Verification items for the finished model (mm, model axes). A direction names the side the tool comes from. Coordinates: 2 decimals unless noted, no trailing zeros. Write each loop counter-clockwise with the first axis right and the second up, starting at its lowest first coordinate (ties: lowest second). Pieces come first, ordered by that corner, then holes. Notation, with made-up numbers: (11, 59.5) - (60, 59.5) arc R12 ccw to (60, 75.5) - close; hole circle Ø11 at (-5.75, -7). An arc over 180 degrees is marked (long way). Use CSV: the item, a comma, the result in double quotes. Start each with the question number.
```python
from build123d import *

# Parameters (mm, degrees)
BOSS_EXTRUDE1_DEPTH = 2.1
SKETCH2_W           = 57.36
SKETCH2_H           = 70
BOSS_EXTRUDE2_DEPTH = 7
SKETCH3_W           = 53.36
SKETCH3_H           = 66
CUT_EXTRUDE1_DEPTH  = 7
SKETCH4_R           = 1.5
CUT_EXTRUDE2_DEPTH  = 2.1
SKETCH6_W           = 40.39
SKETCH6_H           = 2
CUT_EXTRUDE3_DEPTH  = 9.1
BOSS_EXTRUDE3_DEPTH = 9.1
BOSS_EXTRUDE4_DEPTH = 2.1


with BuildPart() as part:
    # Sketch1 → Boss-Extrude1 (new body)
    with BuildSketch(Plane(origin=(0, 0, 0), x_dir=(1, 0, 0), z_dir=(0, 1, 0))):
        Polygon((28.68, 0), (28.68, -8), (28.68, -78), (-28.68, -78), (-28.68, 0), align=None)
    extrude(amount=BOSS_EXTRUDE1_DEPTH)

    # Sketch2 → Boss-Extrude2 (add)
    with BuildSketch(Plane(origin=(0, 2.1, 0), x_dir=(1, 0, 0), z_dir=(0, 1, 0))):
        with Locations((0, -43)):
            Rectangle(SKETCH2_W, SKETCH2_H)
    extrude(amount=BOSS_EXTRUDE2_DEPTH)

    # Sketch3 → Cut-Extrude1 (cut)
    with BuildSketch(Plane(origin=(0, 9.1, 0), x_dir=(1, 0, 0), z_dir=(0, 1, 0))):
        with Locations((0, -43)):
            Rectangle(SKETCH3_W, SKETCH3_H)
    extrude(amount=-CUT_EXTRUDE1_DEPTH, mode=Mode.SUBTRACT)

    # Sketch4 → Cut-Extrude2 (cut)
    with BuildSketch(Plane(origin=(0, 2.1, 0), x_dir=(1, 0, 0), z_dir=(0, 1, 0))):
        with Locations((24.5, -4)):
            Circle(SKETCH4_R)
        with Locations((-24.5, -4)):
            Circle(SKETCH4_R)
    extrude(amount=-CUT_EXTRUDE2_DEPTH, mode=Mode.SUBTRACT)

    # Sketch6 → Cut-Extrude3 (cut)
    with BuildSketch(Plane(origin=(0, 9.1, 0), x_dir=(1, 0, 0), z_dir=(0, 1, 0))):
        with Locations((-6.485, -77)):
            Rectangle(SKETCH6_W, SKETCH6_H)
    extrude(amount=-CUT_EXTRUDE3_DEPTH, mode=Mode.SUBTRACT)

    # Sketch5 → Boss-Extrude3 (add)
    with BuildSketch(Plane(origin=(0, 9.1, 0), x_dir=(1, 0, 0), z_dir=(0, 1, 0))):
        Polygon((-26.68, -76), (-24.14, -76), (-21.6, -78.54), (11.17, -78.54), (13.71, -76), (14.538427125, -76), (14.538427125, -78), (11.998427125, -80.54), (-22.428427125, -80.54), (-24.968427125, -78), (-26.68, -78), align=None)
    extrude(amount=-BOSS_EXTRUDE3_DEPTH)

    # Sketch7 → Boss-Extrude4 (add)
    with BuildSketch(Plane.XZ):
        Polygon((13.71, 76), (-24.14, 76), (-21.6, 78.54), (11.17, 78.54), align=None)
    extrude(amount=-BOSS_EXTRUDE4_DEPTH)


solid = part.part
```
Q1. Gauge pin test, flat ends, axial feed: pin 1 (1.5 mm diameter, centred on x = 4, z = 26.5, fed in from -Y); pin 2 (4.5 mm diameter, centred on x = 23.5, y = 5.5, fed in from +Z); pin 3 (3 mm diameter, centred on x = -10.5, y = 5.5, fed in from -Z); pin 4 (2 mm diameter, centred on x = -3.5, z = 15, fed in from +Y). Record the tip position at first contact, or that the pin passes through.
Q2. Cross-section at C-C (y = 4.75). Record the cut outline in (x, z).
Q3. Scan lines: line 1 along X through (y, z) = (1.45, 4); line 2 along Z through (x, y) = (-2, 8.5); line 3 along Z through (x, y) = (24.5, 1.3). Record each from-to range of solid material in increasing order. Write a range as from..to.
Q4. Release check for a two-part mould opening along Z. For faces 1 (the flat face through (22, 4, 78)), 2 (the flat face through (0, 6, 10)), 3 (the flat face through (0, 6, 8)), 4 (the flat face through (12.42, 5.65, 77.29)) record: released by +Z, released by -Z, zero draft, split by the parting line, or undercut.
Q5. Cross-section at D-D (x = -15.5). Record the cut outline in (y, z).
Q6. Cross-section at A-A (x = 24.5). Record the cut outline in (y, z), plus the area to 4 significant figures.
Q7. Tool access check on faces 5 (the flat face through (0, 2.1, 4)), 6 (the flat face through (-22.89, 5.65, 77.25)), 7 (the flat face through (-27, 5, 78)). Record the directions out of +Z, -Z, +X, -X, +Y, -Y that give a thin tool (end or side, any length) a straight path to the whole face; none if there is none.
Q8. Cross-section at B-B (z = 4). Record the cut outline in (x, y).
Reply:
1,pin 1,"y = 0"
1,pin 2,"z = 78"
1,pin 3,"z = 8"
1,pin 4,"y = 2.1"
2,outline,"(-28.68, 8) - (28.68, 8) - (28.68, 78) - (14.54, 78) - (12, 80.54) - (-22.43, 80.54) - (-24.97, 78) - (-28.68, 78) - close; hole (-26.68, 10) - (26.68, 10) - (26.68, 76) - (13.71, 76) - (11.17, 78.54) - (-21.6, 78.54) - (-24.14, 76) - (-26.68, 76) - close"
3,line 1,"-28.68..-26, -23..23, 26..28.68"
3,line 2,"8..10, 78.54..80.54"
3,line 3,"0..2.5, 5.5..78"
4,face 1,"released by +Z"
4,face 2,"undercut"
4,face 3,"released by -Z"
4,face 4,"undercut"
5,outline,"(0, 0) - (2.1, 0) - (2.1, 8) - (9.1, 8) - (9.1, 10) - (2.1, 10) - (2.1, 78.54) - (9.1, 78.54) - (9.1, 80.54) - (0, 80.54) - close"
6,outline,"(0, 0) - (2.1, 0) - (2.1, 2.5) - (0, 2.5) - close; (0, 5.5) - (2.1, 5.5) - (2.1, 8) - (9.1, 8) - (9.1, 10) - (2.1, 10) - (2.1, 76) - (9.1, 76) - (9.1, 78) - (0, 78) - close"
6,area,"185.5 mm^2"
7,face 5,"-Z, +X, -X, +Y"
7,face 6,"+Y"
7,face 7,"+Z, -X, +Y, -Y"
8,outline,"(-28.68, 0) - (-26, 0) - (-26, 2.1) - (-28.68, 2.1) - close; (-23, 0) - (23, 0) - (23, 2.1) - (-23, 2.1) - close; (26, 0) - (28.68, 0) - (28.68, 2.1) - (26, 2.1) - close"
